from build123d import *

# Parameters (mm, degrees)
F0_W     = 152.4
F0_H     = 152.4
F1_DEPTH = 76.2
F4_DEPTH = 152.401
F5_DEPTH = 152.401


with BuildPart() as f1:
    # F0 (on Top) → F1 (new body, symmetric)
    with BuildSketch(Plane.XY):
        Rectangle(F0_W, F0_H)
    extrude(amount=F1_DEPTH, both=True)

    # F2 (on face) → F4 (cut, through all)
    with BuildSketch(Plane.YZ.offset(76.2)):
        Polygon((-76.2, 76.2), (-76.2, 0), (0, 76.2), align=None)
    extrude(amount=-F4_DEPTH, mode=Mode.SUBTRACT)

    # F3 (on face) → F5 (cut, through all)
    with BuildSketch(Plane.XZ.offset(76.2)):
        Polygon((76.2, 76.2), (0, 76.2), (76.2, 0), align=None)
    extrude(amount=-F5_DEPTH, mode=Mode.SUBTRACT)


solid = f1.part
Check sheet for the modelled part. Datum: model origin and axes. Units: mm. Round coordinates to 2 decimals unless told otherwise and drop trailing zeros. Write each loop counter-clockwise with the first axis right and the second up, starting at its lowest first coordinate (ties: lowest second). Pieces come first, ordered by that corner, then holes. Notation, with made-up numbers: (67.5, -1.75) - (101.5, -1.75) arc R24 cw to (101.5, 25.25) - close; hole circle Ø11 at (29, 67). An arc over 180 degrees is marked (long way). Return JSON: item names as keys, results as strings.
Q1. Cross-section at B-B (y = 38). Record the boundary of the cut face in (x, z), then the cut area to 3 significant figures.
Returned:
{"outline": "(-76.2, -76.2) - (76.2, -76.2) - (76.2, 0) - (0, 76.2) - (-76.2, 76.2) - close", "area": "20,300 mm²"}
Q2. Scan lines: L1, parallel to X at y = -26.5, z = 8.5; L2, parallel to Z at x = 54, y = 38; L3, parallel to Z at x = 37.5, y = 33. Record each from-to range of solid material in increasing order. Write a range as from..to.
Returned:
{"L1": "x = -76.2..67.7", "L2": "z = -76.2..22.2", "L3": "z = -76.2..38.7"}
Q3. Cross-section at A-A (x = 33). Record the boundary of the cut face in (y, z).
Returned:
{"outline": "(-76.2, -76.2) - (76.2, -76.2) - (76.2, 43.2) - (-33, 43.2) - (-76.2, 0) - close"}
Q4. Depth check by flat-ended pin: P1, Ø8, axis at x = -39, y = -19.5, coming from the +Z side; P2, Ø8, axis at x = 1, y = -17, coming from the +Z side. Enter the tip coordinate at first touch or a pass-through.
Returned:
{"P1": "stops at z = 60.7", "P2": "stops at z = 63.2"}
Q5. Cross-section at C-C (z = 18). Record the boundary of the cut face in (x, y), then the cut area to 3 significant figures.
Returned:
{"outline": "(-76.2, -58.2) - (58.2, -58.2) - (58.2, 76.2) - (-76.2, 76.2) - close", "area": "18,100 mm²"}
Q6. Cross-section at D-D (z = 61.5). Record the boundary of the cut face in (x, y), then the cut area to 3 significant figures.
Returned:
{"outline": "(-76.2, -14.7) - (14.7, -14.7) - (14.7, 76.2) - (-76.2, 76.2) - close", "area": "8,260 mm²"}
